```python
from build123d import *

# Parameters (mm, degrees)
SKETCH1_W           = 2000
SKETCH1_H           = 1000
BOSS_EXTRUDE1_DEPTH = 150
SKETCH2_W           = 304.8
SKETCH2_H           = 1000
BOSS_EXTRUDE2_DEPTH = 10
SKETCH3_R           = 25.4
CUT_EXTRUDE1_DEPTH  = 161


with BuildPart() as part:
    # Sketch1 → Boss-Extrude1 (new body)
    with BuildSketch(Plane(origin=(0, 0, 0), x_dir=(1, 0, 0), z_dir=(0, 1, 0))):
        Rectangle(SKETCH1_W, SKETCH1_H)
    extrude(amount=BOSS_EXTRUDE1_DEPTH)

    # Sketch2 → Boss-Extrude2 (add)
    with BuildSketch(Plane(origin=(0, 150, 0), x_dir=(1, 0, 0), z_dir=(0, 1, 0))):
        with Locations((847.6, 0)):
            Rectangle(SKETCH2_W, SKETCH2_H)
    extrude(amount=BOSS_EXTRUDE2_DEPTH)

    # Sketch3 → Cut-Extrude1 (cut, through all)
    with BuildSketch(Plane.XZ):
        with Locations((403.1, 254)):
            Circle(SKETCH3_R)
        with Locations((403.1, -254)):
            Circle(SKETCH3_R)
    extrude(amount=-CUT_EXTRUDE1_DEPTH, mode=Mode.SUBTRACT)


solid = part.part
```
Work out the finished part from the listing and answer in its coordinate system (mm). A direction names the side the tool comes from. Coordinates: 2 decimals unless noted, no trailing zeros. Write each loop counter-clockwise with the first axis right and the second up, starting at its lowest first coordinate (ties: lowest second). Pieces come first, ordered by that corner, then holes. Notation, with made-up numbers: (47, 29.5) - (57, 29.5) arc R12 ccw to (57, 43.5) - close; hole circle Ø11 at (-25.5, -16). An arc over 180 degrees is marked (long way). Answer as a JSON object with one key per item and string values.
Q1. Consider L1, parallel to Z at x = 403.1, y = 85; L2, parallel to Y at x = -851.5, z = 233. Determine where each line is inside the solid, lowest interval first. Write a range as from..to.
Results list:
{"L1": "z = -500..-279.4, -228.6..228.6, 279.4..500", "L2": "y = 0..150"}
Q2. Given pin 1 Ø10 at (x, z) = (-459.5, -17) entering from +Y, flat-ended and moving along its own axis, determine where the tip first touches the part or whether it passes through.
Results list:
{"pin 1": "stops at y = 150"}
Q3. Find section B-B (z = 132). Write down the section's boundary in (x, y), plus the area to 3 significant figures.
Results list:
{"outline": "(-1000, 0) - (1000, 0) - (1000, 160) - (695.2, 160) - (695.2, 150) - (-1000, 150) - close", "area": "303,000 mm^2"}
Q4. Find section C-C (x = 191.5). Write down the section's boundary in (y, z).
Results list:
{"outline": "(0, -500) - (150, -500) - (150, 500) - (0, 500) - close"}
Q5. For a pull along Z with two mould halves and no side action, classify faces 1 (the cylindrical face through (382.943, 73.95, 238.544)), 2 (the flat face through (1000, 79, 7)), 3 (the flat face through (-14, 79, -500)) as pulls with the +Z half, pulls with the -Z half, needs draft (parallel to the pull), parting line crosses it, or undercut.
Results list:
{"face 1": "undercut", "face 2": "needs draft", "face 3": "pulls with the -Z half"}
Q6. Which of the six approach directions +Z, -Z, +X, -X, +Y, -Y give full straight-line access (tool end or side, diameter ignored) to faces 4 (the flat face through (-164, 150, -7)), 5 (the cylindrical face through (382.943, 73.95, -269.456))?
Results list:
{"face 4": "+Z, -Z, -X, +Y", "face 5": "+Y, -Y"}
Q7. Find section A-A (z = -254). Write down the section's boundary in (x, y), plus the area to 3 significant figures.
Results list:
{"outline": "(-1000, 0) - (377.7, 0) - (377.7, 150) - (-1000, 150) - close; (428.5, 0) - (1000, 0) - (1000, 160) - (695.2, 160) - (695.2, 150) - (428.5, 150) - close", "area": "295,000 mm^2"}
